```python
from build123d import *

# Parameters (mm, degrees)
F1_DEPTH = 25.4
F2_DEPTH = 12.7
F3_W     = 15.489865
F3_H     = 12.7
F4_DEPTH = 6.35


with BuildPart() as f1:
    # F0 (on Right) → F1 (new body)
    with BuildSketch(Plane.YZ):
        Polygon((-25.4, 0), (0, 0), (0, 31.75), (-12.7, 31.75), (-12.7, 12.7), (-25.4, 12.7), align=None)
    extrude(amount=F1_DEPTH)

    # F1_face (on face) → F2 (join)
    with BuildSketch(Plane(origin=(25.4, -9.978571, 13.153571), x_dir=(0, 1, 0), z_dir=(1, 0, 0))):
        Polygon((-15.421429, -13.153571), (9.978571, -13.153571), (9.978571, 18.596429), (-2.721429, 18.596429), (-2.721429, -0.453571), (-15.421429, -0.453571), align=None)
    extrude(amount=F2_DEPTH)

    # F3 (on face) → F4 (cut)
    with BuildSketch(Plane.XY.offset(31.75)):
        with Locations((18.207432, -6.35)):
            Rectangle(F3_W, F3_H)
    extrude(amount=-F4_DEPTH, mode=Mode.SUBTRACT)


solid = f1.part
```
Part model, mm, in its own coordinate system. A direction names the side the tool comes from. Round coordinates to 2 decimals unless told otherwise and drop trailing zeros. Loops run counter-clockwise (first coordinate to the right, second up) from the corner with the lowest first, then second, coordinate; pieces in that order, holes last. Notation, with made-up numbers: (49, -15) -> (81, -15) arc R26 cw to (81, 6) -> close; hole circle Ø3 at (26, -36.75). An arc over 180 degrees is marked (long way). Use one line per item in the form item = value. Start each with the question number.
Item 1: Band-saw the part on B-B (x = 17). List the corners of the cut face in (y, z).
Item 2: Drill centre lines: line 1 along X through (y, z) = (-6.25, 30); line 2 along Z through (x, y) = (23, -12); line 3 along Y through (x, z) = (14, 21.5). Where is each one in solid material? Low to high.
Item 3: Band-saw the part on D-D (x = 28). List the corners of the cut face in (y, z), plus the area to 3 significant figures.
Item 4: Tool access for faces 1 (the flat face through (19, -19, 12.7)), 2 (the flat face through (19, -25.4, 6)), 3 (the flat face through (25.952, -6, 29)): list every direction of +Z, -Z, +X, -X, +Y, -Y with a clear straight run to the whole face (end or side of a thin tool).
Item 5: Band-saw the part on A-A (y = -7.5). List the corners of the cut face in (x, z), plus the area to 3 significant figures.
Item 6: Drop flat-ended pins along their axis: pin 1 Ø10 at (x, y) = (15, -19.5) entering from +Z; pin 2 Ø9.5 at (x, z) = (26.5, 24.5) entering from -Y; pin 3 Ø7 at (y, z) = (-8, 28) entering from -X; pin 4 Ø8 at (x, y) = (20, -14) entering from +Z. Give the stop position or say it passes through.
Item 7: Band-saw the part on C-C (z = 21). List the corners of the cut face in (x, y), plus the area to 3 significant figures.
Item 8: Two-plate mould, pull along X, no slides. Class faces 4 (the flat face through (19, -13, 0)), 5 (the flat face through (38.1, -10, 13)), 6 (the flat face through (18, -6, 25.4)), 7 (the flat face through (10.462, -6, 29)): released by +X, released by -X, zero draft, split by the parting line, or undercut.
Data:
q1.outline = (-25.4, 0) -> (0, 0) -> (0, 25.4) -> (-12.7, 25.4) -> (-12.7, 12.7) -> (-25.4, 12.7) -> close
q2.line_1 = 0 to 10.46, 25.95 to 38.1
q2.line_2 = 0 to 25.4
q2.line_3 = -12.7 to 0
q3.outline = (-25.4, 0) -> (0, 0) -> (0, 31.75) -> (-12.7, 31.75) -> (-12.7, 12.7) -> (-25.4, 12.7) -> close
q3.area = 565 mm^2
q4.face_1 = +Z, +X, -X, -Y
q4.face_2 = +Z, -Z, +X, -X, -Y
q4.face_3 = +Z, +Y, -Y
q5.outline = (0, 0) -> (38.1, 0) -> (38.1, 31.75) -> (25.95, 31.75) -> (25.95, 25.4) -> (10.46, 25.4) -> (10.46, 31.75) -> (0, 31.75) -> close
q5.area = 1,110 mm^2
q6.pin_1 = 12.7
q6.pin_2 = -12.7
q6.pin_3 = 0
q6.pin_4 = 25.4
q7.outline = (0, -12.7) -> (38.1, -12.7) -> (38.1, 0) -> (0, 0) -> close
q7.area = 484 mm^2
q8.face_4 = zero draft
q8.face_5 = released by +X
q8.face_6 = undercut
q8.face_7 = undercut
